Part model, mm, in its own coordinate system. Face numbers are marked on the shaded views. Round coordinates to 2 decimals unless told otherwise and drop trailing zeros. Write each loop counter-clockwise with the first axis right and the second up, starting at its lowest first coordinate (ties: lowest second). Pieces come first, ordered by that corner, then holes. Notation, with made-up numbers: M 69,15 L 102,15 A24 ccw 102,39 Z; hole C 55.25,51 d10. An arc over 180 degrees is marked long. Use one line per item in the form item = value. Start each with the question number.
Item 1: Flat gauge pins, fed straight in: pin 1 Ø0.6 at (y, z) = (-66.5, 16.5) entering from +X; pin 2 Ø5 at (x, y) = (3, -56.5) entering from -Z; pin 3 Ø8 at (x, z) = (12, 12.5) entering from +Y; pin 4 Ø1.8 at (x, y) = (12, -66.5) entering from -Z. Where does each tip first touch, or does it go through?
Item 2: Cut at C-C, the plane z = -24. Give the cut face in (x, y), then the cut area to 3 significant figures.
Item 3: Cut at A-A, the plane z = -37. Give the cut face in (x, y).
Item 4: Cut at B-B, the plane x = 8.25. Give the cut face in (y, z), then the cut area to 3 significant figures.
Item 5: Probe L1, parallel to Y at x = 1, z = 15.5; L2, parallel to Z at x = 9, y = -67; L3, parallel to X at y = -58.25, z = 33. List the from-to ranges inside material, lowest first.
Item 6: Mould opens along Z. For the marked faces 1 and 2 say: +Z half, -Z half, draft (parallel to the pull), parting line (faces both ways), or undercut.
Item 7: Cut at D-D, the plane x = 2. State how many separate pieces and enclosed holes the cut face has, then the cut area to 3 significant figures.
from build123d import *

# Parameters (mm, degrees)
SKETCH_1_R      = 0.978970723
SKETCH_1_R_2    = 1.00064107
EXTRUDE_1_DEPTH = 4.5
SKETCH_2_R      = 0.95
EXTRUDE_2_DEPTH = 11.76992
FILLET_1_R      = 2
FILLET_2_R      = 0.8


with BuildPart() as part:
    # 草图1 → 凸台-拉伸1 (new body)
    with BuildSketch(Plane(origin=(0, 0, 0), x_dir=(0, 0, -1), z_dir=(1, 0, 0))):
        with BuildLine():
            Line((-39.321623093, -59.770803947), (-31.880209784, -65.026985305))
            Line((-31.880209784, -65.026985305), (-28.883499317, -68.026462319))
            Line((-28.883499317, -68.026462319), (3.215977086, -68.026462319))
            Line((3.215977086, -68.026462319), (55.639850151, -60.599346768))
            ThreePointArc((55.639850151, -60.599346768), (57.197718569, -61.373971566), (58.88034135, -60.931503307))
            Line((58.88034135, -60.931503307), (58.88034135, -56.894014776))
            ThreePointArc((58.88034135, -56.894014776), (57.069785986, -56.468040051), (55.474117274, -57.423763105))
            Line((55.474117274, -57.423763105), (2.519577321, -52.531922747))
            Line((2.519577321, -52.531922747), (0.064241127, -48.627089366))
            Line((0.064241127, -48.627089366), (-28.81990203, -48.627089366))
            Line((-28.81990203, -48.627089366), (-34.57208033, -56.689800145))
            Line((-34.57208033, -56.689800145), (-39.321623093, -59.770803947))
        make_face()
        with Locations((-0.389382662, -58.037544978)):
            Circle(SKETCH_1_R, mode=Mode.SUBTRACT)
        with Locations((-28.381009123, -58.037544978)):
            Circle(SKETCH_1_R_2, mode=Mode.SUBTRACT)
        Polygon((-26.120321367, -51.538768317), (-26.120321367, -64.493439573), (-2.641506603, -64.493439573), (-2.630422679, -51.527089366), align=None, mode=Mode.SUBTRACT)
        Polygon((3.119577321, -56.086889198), (3.119577321, -64.024429188), (38.403692816, -60.533510862), align=None, mode=Mode.SUBTRACT)
        Polygon((-31.880209784, -57.326749532), (-31.880422679, -62.379599563), (-35.223651542, -60.515120464), align=None, mode=Mode.SUBTRACT)
    extrude(amount=EXTRUDE_1_DEPTH)

    # 草图2 → 凸台-拉伸2 (add)
    with BuildSketch(Plane(origin=(4.5, 0, 0), x_dir=(0, 0, -1), z_dir=(1, 0, 0))):
        Polygon((-25.62686112, -68.026462319), (-25.620633929, -64.493439573), (-13.620633929, -64.493439573), (-13.620633929, -68.026462319), align=None)
        with Locations((-22.620633929, -66.317445767)):
            Circle(SKETCH_2_R, mode=Mode.SUBTRACT)
        with Locations((-16.620633929, -66.317445767)):
            Circle(SKETCH_2_R, mode=Mode.SUBTRACT)
    extrude(amount=EXTRUDE_2_DEPTH)

    # 圆角1
    # the kernel refuses this fillet: 2 mm, written as the material it adds along each edge
    with BuildSketch(Plane(origin=(0, -56.689800145, 34.57208033), x_dir=(0, -0.5442183706519984, 0.8389436006340856), z_dir=(1, 0, 0))) as fillet_1_piece_1:
        with BuildLine():
            CenterArc((FILLET_1_R * 0.19006878131, -FILLET_1_R), FILLET_1_R, 90, 21.523541221)
            Line((-FILLET_1_R * 0.176814696818, -FILLET_1_R * 0.0697330955707), (0, 0))
            Line((0, 0), (FILLET_1_R * 0.19006878131, 0))
        make_face()
    extrude(amount=4.5)
    with BuildSketch(Plane(origin=(0, -52.531922747, -2.519577321), x_dir=(0, -0.09198645148038477, -0.9957602586687455), z_dir=(1, 0, 0))) as fillet_1_piece_2:
        with BuildLine():
            CenterArc((FILLET_1_R * 0.493803738743, FILLET_1_R), FILLET_1_R, 217.439335715, 52.560664285)
            Line((-FILLET_1_R * 0.30019370817, FILLET_1_R * 0.392078907838), (0, 0))
            Line((0, 0), (FILLET_1_R * 0.493803738743, 0))
        make_face()
    extrude(amount=4.5)
    with BuildSketch(Plane(origin=(4.5, -64.493439573, 13.620633929), x_dir=(0, 0, -1), z_dir=(0, -1, 0))) as fillet_1_piece_3:
        with BuildLine():
            CenterArc((FILLET_1_R, FILLET_1_R), FILLET_1_R, 180, 90)
            Line((0, FILLET_1_R), (0, 0))
            Line((0, 0), (FILLET_1_R, 0))
        make_face()
    extrude(amount=3.533022746)
    with BuildSketch(Plane(origin=(4.5, -73.026454553, 25.635673944), x_dir=(0, 0.0017625646835904966, 0.9999984466816618), z_dir=(0, 0.9999984466816617, -0.0017625646835904966))) as fillet_1_piece_4_section:
        with BuildLine():
            CenterArc((FILLET_1_R, FILLET_1_R), FILLET_1_R, 180, 90)
            Line((0, FILLET_1_R), (0, 0))
            Line((0, 0), (FILLET_1_R, 0))
        make_face()
    fillet_1_piece_4 = extrude(amount=13.533028234, mode=Mode.PRIVATE)
    fillet_1_piece_4 = split(fillet_1_piece_4, bisect_by=Plane(origin=(4.696560989, -68.026462319, 26.482181103), z_dir=(0, 1, 0)), keep=Keep.TOP, mode=Mode.PRIVATE)
    fillet_1_piece_4 = split(fillet_1_piece_4, bisect_by=Plane(origin=(4.696560989, -64.493439573, 26.482181103), z_dir=(0, -1, 0)), keep=Keep.TOP, mode=Mode.PRIVATE)
    add(fillet_1_piece_4)
    # the kernel refuses this fillet: 2 mm, written as the material it takes off along each edge
    with BuildSketch(Plane(origin=(-2.574882543, -48.627089366, 28.81990203), x_dir=(0, 0, -1), z_dir=(1, 0, 0))) as fillet_1_2_piece_1:
        with BuildLine():
            CenterArc((FILLET_1_R * 0.514976508546, -FILLET_1_R), FILLET_1_R, 90, 54.49480721)
            Line((-FILLET_1_R * 0.299086376608, -FILLET_1_R * 0.419223262333), (0, 0))
            Line((0, 0), (FILLET_1_R * 0.514976508546, 0))
        make_face()
    extrude(amount=9.649765085, mode=Mode.SUBTRACT)
    with BuildSketch(Plane(origin=(-2.762343959, -48.627089366, -0.064241127), x_dir=(0, -0.8465516071687306, -0.532306656355187), z_dir=(1, 0, 0))) as fillet_1_2_piece_2:
        with BuildLine():
            CenterArc((FILLET_1_R * 0.552468791842, -FILLET_1_R), FILLET_1_R, 90, 57.83856081)
            Line((-FILLET_1_R * 0.294082815326, -FILLET_1_R * 0.467693343645), (0, 0))
            Line((0, 0), (FILLET_1_R * 0.552468791842, 0))
        make_face()
    extrude(amount=10.024687918, mode=Mode.SUBTRACT)
    with BuildSketch(Plane(origin=(-2.072419305, -68.026462319, 28.883499317), x_dir=(0, 0.7074329539484039, 0.70678045789894), z_dir=(1, 0, 0))) as fillet_1_2_piece_3:
        with BuildLine():
            CenterArc((FILLET_1_R * 0.414483860929, -FILLET_1_R), FILLET_1_R, 90, 45.026435379)
            Line((-FILLET_1_R * 0.292949093019, -FILLET_1_R * 0.293219542101), (0, 0))
            Line((0, 0), (FILLET_1_R * 0.414483860929, 0))
        make_face()
    extrude(amount=8.644838609, mode=Mode.SUBTRACT)
    with BuildSketch(Plane(origin=(-7.384077235, -59.770803947, 39.321623093), x_dir=(0, -0.5769336472143782, -0.816791017771324), z_dir=(1, 0, 0))) as fillet_1_2_piece_4:
        with BuildLine():
            CenterArc((FILLET_1_R * 1.47681544699, FILLET_1_R), FILLET_1_R, 158.206425449, 111.793574551)
            Line((FILLET_1_R * 0.548287978811, FILLET_1_R * 1.37126370795), (0, 0))
            Line((0, 0), (FILLET_1_R * 1.47681544699, 0))
        make_face()
    extrude(amount=19.26815447, mode=Mode.SUBTRACT)

    # 圆角2
    fillet_2_edges = [part.edges().sort_by_distance(p)[0] for p in [
        (2.25, -56.894014776, -58.88034135),
        (2.25, -60.931503307, -58.88034135),
        (2.25, -51.527089366, 2.630422679),
        (2.25, -51.538768317, 26.120321367),
        (2.25, -64.493439573, 26.120321367),
        (2.25, -64.493439573, 2.641506603),
        (2.25, -56.086889198, -3.119577321),
        (2.25, -64.024429188, -3.119577321),
    ]]
    fillet(fillet_2_edges, radius=FILLET_2_R)


solid = part.part
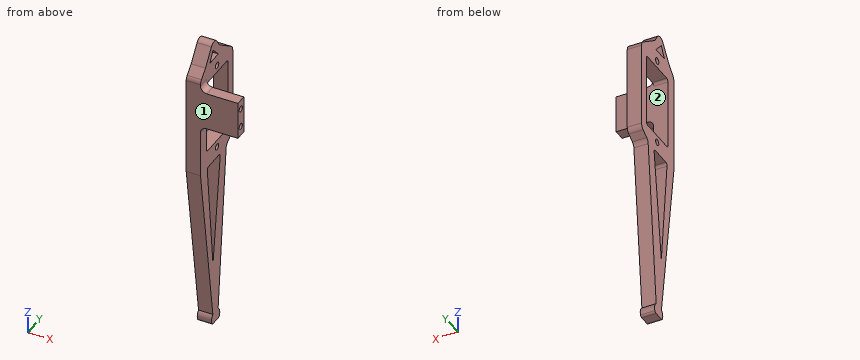
Model answer:
q1.pin_1 = 4.5
q1.pin_2 = -58.88
q1.pin_3 = -64.49
q1.pin_4 = 13.62
q2.outline = M 0,-65.08 L 4.5,-65.08 L 4.5,-61.96 L 0,-61.96 Z; M 0,-58.72 L 4.5,-58.72 L 4.5,-54.52 L 0,-54.52 Z
q2.area = 33.0 mm²
q3.outline = M 0,-63.24 L 4.5,-63.24 L 4.5,-60.67 L 0,-60.67 Z; M 0,-60.36 L 4.5,-60.36 L 4.5,-55.72 L 0,-55.72 Z
q4.outline = M -68.03,13.62 L -64.49,13.62 L -64.49,25.62 L -68.03,25.63 Z; hole C -66.32,16.62 d1.9; hole C -66.32,22.62 d1.9
q4.area = 36.7 mm²
q5.L1 = -68.03 to -64.49, -51.53 to -48.63
q5.L2 = 13.62 to 15.96, 17.28 to 21.96, 23.28 to 25.63
q5.L3 = 0 to 4.5
q6.face_1 = draft
q6.face_2 = undercut
q7.separate_pieces = 1
q7.enclosed_holes = 5
q7.area = 744 mm²
